The model under review builds one solid part; all positions refer to its coordinate system, in mm. A direction names the side the tool comes from. Coordinates: 2 decimals unless noted, no trailing zeros. Write each loop counter-clockwise with the first axis right and the second up, starting at its lowest first coordinate (ties: lowest second). Pieces come first, ordered by that corner, then holes.
1) Add section A-A, the plane z = 5.45. Give the number of separate pieces and of enclosed holes in the cut face, then the cut area to 3 significant figures.
2) Add section B-B, the plane y = -1.25. State the section outline as (x, z) points, then the cut area to 3 significant figures.
3) Add section D-D, the plane y = 4.25. State the section outline as (x, z) points.
4) For line 1 (X direction, y = -5.5, z = 5.7); line 2 (X direction, y = 0, z = 4.65); line 3 (X direction, y = -5, z = 4.7), list the stretches that pass through material, from the lowest coordinate up.
5) Add section C-C, the plane x = -21.75. State the section outline as (y, z) points, then the cut area to 3 significant figures.
6) For P1, Ø2, axis at x = -13.5, z = 3, coming from the +Y side; P2, Ø1.5, axis at x = -22.5, z = 4.5, coming from the +Y side; P3, Ø0.8, axis at x = -22, y = -3.5, coming from the +Z side, all flat-tipped, find the tip position at first contact; note any pin that passes through.
7) Machinability: for faces 4 (the flat face through (-15, -5, 4)), 5 (the flat face through (-18, -2, 6)), which of the approach directions +Z, -Z, +X, -X, +Y, -Y give a long, thin tool a straight path to every point of the face, cutting with its end or side? Answer none if there is none.
8) Mouldability with a two-part tool opening along X and no side actions: class faces 1 (the flat face through (-22, -3, 4)), 2 (the cylindrical face through (-19.47, -9.238, 2.958)), 3 (the flat face through (-18, -2, 0)) as released by +X, released by -X, zero draft, split by the parting line, or undercut.
from build123d import *

# Parameters (mm, degrees)
SKETCH2_R           = 7.5
BOSS_EXTRUDE1_DEPTH = 6
SKETCH3_R           = 6.5
SKETCH3_R_2         = 5.5
CUT_EXTRUDE1_DEPTH  = 2
SKETCH4_R           = 0.75
CUT_EXTRUDE2_DEPTH  = 2


with BuildPart() as part:
    # Sketch2 → Boss-Extrude1 (new body)
    with BuildSketch(Plane.XY):
        with Locations((-17.844062558, -1.916140946)):
            Circle(SKETCH2_R)
    extrude(amount=BOSS_EXTRUDE1_DEPTH)

    # Sketch3 → Cut-Extrude1 (cut)
    with BuildSketch(Plane.XY.offset(6)):
        with Locations((-17.844062558, -1.916140946)):
            Circle(SKETCH3_R)
        with Locations((-17.844062558, -1.916140946)):
            Circle(SKETCH3_R_2, mode=Mode.SUBTRACT)
    extrude(amount=-CUT_EXTRUDE1_DEPTH, mode=Mode.SUBTRACT)

    # Sketch4 → Cut-Extrude2 (cut)
    with BuildSketch(Plane.XY.offset(6)):
        with Locations((-17.844062558, 0.583859054)):
            Circle(SKETCH4_R)
        with Locations((-15.678999049, -3.166140946)):
            Circle(SKETCH4_R)
        with Locations((-20.009126068, -3.166140946)):
            Circle(SKETCH4_R)
        with Locations((-21.542818561, 0.177111078)):
            Circle(SKETCH4_R)
        with Locations((-18.513628873, 2.280784232)):
            Circle(SKETCH4_R)
        with Locations((-14.980242093, 1.224087126)):
            Circle(SKETCH4_R)
        with Locations((-13.603370535, -2.197265767)):
            Circle(SKETCH4_R)
        with Locations((-15.419826565, -5.406925936)):
            Circle(SKETCH4_R)
        with Locations((-19.061781743, -5.987953808)):
            Circle(SKETCH4_R)
        with Locations((-21.786769538, -3.502823545)):
            Circle(SKETCH4_R)
    extrude(amount=-CUT_EXTRUDE2_DEPTH, mode=Mode.SUBTRACT)


solid = part.part
Geometry results:
1. separate pieces: 2
1. enclosed holes: 11
1. area: 121 mm2
2. outline: (-25.31, 0) - (-10.37, 0) - (-10.37, 6) - (-11.38, 6) - (-11.38, 4) - (-12.38, 4) - (-12.38, 6) - (-23.3, 6) - (-23.3, 4) - (-24.31, 4) - (-24.31, 6) - (-25.31, 6) - close
2. area: 85.6 mm2
3. outline: (-22.11, 0) - (-13.57, 0) - (-13.57, 6) - (-15.79, 6) - (-15.79, 4) - (-19.9, 4) - (-19.9, 6) - (-22.11, 6) - close
4. line 1: x = -24.43 to -23.27, -22.02 to -19.63, -18.49 to -16.16, -14.68 to -13.67, -12.42 to -11.26
4. line 2: x = -25.1 to -24.06, -23 to -22.27, -20.81 to -18.31, -17.37 to -12.69, -11.63 to -10.59
4. line 3: x = -24.68 to -23.57, -22.4 to -16.05, -14.79 to -13.29, -12.12 to -11.01
5. outline: (-8.32, 0) - (4.49, 0) - (4.49, 6) - (3.28, 6) - (3.28, 4) - (1.96, 4) - (1.96, 6) - (0.9, 6) - (0.9, 4) - (-0.54, 4) - (-0.54, 6) - (-2.75, 6) - (-2.75, 4) - (-4.25, 4) - (-4.25, 6) - (-5.79, 6) - (-5.79, 4) - (-7.11, 4) - (-7.11, 6) - (-8.32, 6) - close
5. area: 65.7 mm2
6. P1: stops at y = 4.8
6. P2: stops at y = 4.49
6. P3: stops at z = 4
7. face 4: +Z
7. face 5: +Z, +X, -X, +Y, -Y
8. face 1: undercut
8. face 2: split by the parting line
8. face 3: zero draft
